from build123d import *

# Parameters (mm, degrees)
SKETCH1_W           = 20.9
SKETCH1_H           = 12
BOSS_EXTRUDE1_DEPTH = 6.3
SKETCH2_R           = 4
BOSS_EXTRUDE2_DEPTH = 5
SKETCH3_R           = 2.5
CUT_EXTRUDE1_DEPTH  = 11.3


with BuildPart() as part:
    # Sketch1 → Boss-Extrude1 (new body)
    with BuildSketch(Plane(origin=(0, 0, 0), x_dir=(1, 0, 0), z_dir=(0, 1, 0))):
        Rectangle(SKETCH1_W, SKETCH1_H)
    extrude(amount=BOSS_EXTRUDE1_DEPTH)

    # Sketch2 → Boss-Extrude2 (add)
    with BuildSketch(Plane(origin=(0, 6.3, 0), x_dir=(1, 0, 0), z_dir=(0, 1, 0))):
        with Locations((-4.45, 0)):
            Circle(SKETCH2_R)
        with Locations((4.45, 0)):
            Circle(SKETCH2_R)
    extrude(amount=BOSS_EXTRUDE2_DEPTH)

    # Sketch3 → Cut-Extrude1 (cut)
    with BuildSketch(Plane(origin=(0, 11.3, 0), x_dir=(1, 0, 0), z_dir=(0, 1, 0))):
        with Locations((4.45, 0)):
            Circle(SKETCH3_R)
        with Locations((-4.45, 0)):
            Circle(SKETCH3_R)
    extrude(amount=-CUT_EXTRUDE1_DEPTH, mode=Mode.SUBTRACT)


solid = part.part
Design review of the part built by this model. Coordinates are the model's own, in mm. A direction names the side the tool comes from. Give positions to 0.01 mm unless a question says otherwise; leave off trailing zeros. Loops run counter-clockwise (first coordinate to the right, second up) from the corner with the lowest first, then second, coordinate; pieces in that order, holes last. Notation, with made-up numbers: M 70,65.25 L 110,65.25 A16 cw 110,92.25 Z; hole C -28.5,13 d3. An arc over 180 degrees is marked long. Answer as a JSON object with one key per item and string values.
Item 1: We need section C-C (z = 0). State the section outline as (x, y) points, and give its area (3 significant figures).
Output values:
{"outline": "M -10.45,0 L -6.95,0 L -6.95,11.3 L -8.45,11.3 L -8.45,6.3 L -10.45,6.3 Z; M -1.95,0 L 1.95,0 L 1.95,11.3 L 0.45,11.3 L 0.45,6.3 L -0.45,6.3 L -0.45,11.3 L -1.95,11.3 Z; M 6.95,0 L 10.45,0 L 10.45,6.3 L 8.45,6.3 L 8.45,11.3 L 6.95,11.3 Z", "area": "98.7 mm2"}
Item 2: We need section A-A (x = -4.45). State the section outline as (y, z) points.
Output values:
{"outline": "M 0,-6 L 6.3,-6 L 6.3,-4 L 11.3,-4 L 11.3,-2.5 L 0,-2.5 Z; M 0,2.5 L 11.3,2.5 L 11.3,4 L 6.3,4 L 6.3,6 L 0,6 Z"}
Item 3: For P1, Ø1.5, axis at x = 0, y = 8.5, coming from the -Z side; P2, Ø6, axis at x = 4.45, z = 0, coming from the +Y side, all flat-tipped, find the tip position at first contact; note any pin that passes through.
Output values:
{"P1": "stops at z = -1.52", "P2": "stops at y = 11.3"}
Item 4: We need section D-D (y = 1.75). State the section outline as (x, z) points.
Output values:
{"outline": "M -10.45,-6 L 10.45,-6 L 10.45,6 L -10.45,6 Z; hole C -4.45,0 d5; hole C 4.45,0 d5"}
Item 5: We need section B-B (y = 7.5). State the section outline as (x, z) points, and give its area (3 significant figures).
Output values:
{"outline": "C -4.45,0 d8; C 4.45,0 d8; hole C -4.45,0 d5; hole C 4.45,0 d5", "area": "61.3 mm2"}
Item 6: Wall thickness on line 1 along X through (y, z) = (4, 0); line 2 along X through (y, z) = (7.75, 0); line 3 along Z through (x, y) = (-4.45, 7.5): over which ranges is each line inside the solid? List them lowest first.
Output values:
{"line 1": "x = -10.45 to -6.95, -1.95 to 1.95, 6.95 to 10.45", "line 2": "x = -8.45 to -6.95, -1.95 to -0.45, 0.45 to 1.95, 6.95 to 8.45", "line 3": "z = -4 to -2.5, 2.5 to 4"}
Item 7: Mouldability with a two-part tool opening along X and no side actions: class faces 1 (the face through (10.45, 3, 0)), 2 (the face through (4, 11.3, 3)), 3 (the face through (3.583, 8.765, 3.905)) as pulls with the +X half, pulls with the -X half, needs draft (parallel to the pull), parting line crosses it, or undercut.
Output values:
{"face 1": "pulls with the +X half", "face 2": "needs draft", "face 3": "undercut"}
Item 8: Machinability: for faces 4 (the face through (0, 6.3, 0)), 5 (the face through (0, 3, 6)), which of the approach directions +Z, -Z, +X, -X, +Y, -Y give a long, thin tool a straight path to every point of the face, cutting with its end or side? Answer none if there is none.
Output values:
{"face 4": "+Y", "face 5": "+Z, +X, -X, +Y, -Y"}
